Model file for the job. Use its own axes, mm. A direction names the side the tool comes from. Round coordinates to 2 decimals unless told otherwise and drop trailing zeros. Order: outer loops, then holes, each group sorted by start corner. A loop starts at its lowest first (then second) coordinate and runs counter-clockwise, first axis right, second up. Notation, with made-up numbers: (81, 14) -> (106, 14) arc R4 ccw to (106, 19) -> close; hole circle Ø3 at (25.5, -32). An arc over 180 degrees is marked (long way). Put each result on its own line as item: value. Start each with the question number.
Q1. Cut at B-B, the plane x = 10. List the corners of the cut face in (y, z).
Q2. Probe L1, parallel to Y at x = 12, z = 10.25; L2, parallel to X at y = -20.5, z = 5.5; L3, parallel to Y at x = 0.7, z = 6. List the from-to ranges inside material, lowest first.
Q3. Cut at D-D, the plane y = -15.5. List the corners of the cut face in (x, z).
Q4. 3-axis set-ups, long thin cutter, end or side, ignore diameter. For faces 4 (the face through (8.1, -0.5, 0)), 5 (the face through (1, -18, 6)): which of +Z, -Z, +X, -X, +Y, -Y reach the whole face in a straight line?
Q5. Cut at C-C, the plane z = 3.8. List the corners of the cut face in (x, y).
Q6. Cut at A-A, the plane y = -10. List the corners of the cut face in (x, z), and give its area (3 significant figures).
Q7. Pull direction Z, two halves, no side cores. Call faces 1 (the face through (8.1, -0.5, 12)), 2 (the face through (0.493, -11.464, 3.475)), 3 (the face through (18, -1, 6)): released by +Z, released by -Z, zero draft, split by the parting line, or undercut.
Q8. Flat gauge pins, fed straight in: P1, Ø6, axis at x = 21, z = 5, coming from the -Y side; P2, Ø4, axis at y = -10, z = 2.5, coming from the +X side; P3, Ø3, axis at y = -22, z = 2.5, coming from the -X side. Where does each tip first touch, or does it go through?
from build123d import *

# Parameters (mm, degrees)
EXTRUDE_1_DEPTH     = 12
FILLET_1_R          = 6
FILLET_2_R          = 2
FILLET_3_R          = 0.5
SKETCH_2_R          = 1.5
CUT_EXTRUDE_1_DEPTH = 51.931326313
SKETCH_3_R          = 1.5
CUT_EXTRUDE_2_DEPTH = 51.931326313


with BuildPart() as part:
    # 草图1 → 凸台-拉伸1 (new body)
    with BuildSketch(Plane.XY):
        Polygon((0, 0), (35, 0), (35, -1), (1, -1), (1, -35), (0, -35), align=None)
    extrude(amount=EXTRUDE_1_DEPTH)

    # 圆角1
    fillet_1_edges = [part.edges().sort_by_distance(p)[0] for p in [
        (0.5, -35, 12),
        (0.5, -35, 0),
        (35, -0.5, 0),
        (35, -0.5, 12),
    ]]
    fillet(fillet_1_edges, radius=FILLET_1_R - 0.0001)  # a hair under: the kernel refuses the full size

    # 圆角2
    fillet_2_edges = [part.edges().sort_by_distance(p)[0] for p in [
        (0, 0, 6),
    ]]
    fillet(fillet_2_edges, radius=FILLET_2_R)

    # 圆角3
    fillet_3_edges = [part.edges().sort_by_distance(p)[0] for p in [
        (1, -1, 6),
    ]]
    fillet(fillet_3_edges, radius=FILLET_3_R)

    # 草图2 → 切除-拉伸1 (cut, through all)
    with BuildSketch(Plane.ZY):
        with Locations((6, -29)):
            Circle(SKETCH_2_R)
        with Locations((3.8, -10)):
            Circle(SKETCH_2_R)
    extrude(amount=-CUT_EXTRUDE_1_DEPTH, mode=Mode.SUBTRACT)

    # 草图3 → 切除-拉伸2 (cut, through all)
    with BuildSketch(Plane(origin=(0, 0, 0), x_dir=(1, 0, 0), z_dir=(0, 1, 0))):
        with Locations(Location((29, -6, 0), (0, 0, 270))):
            Circle(SKETCH_3_R)
        with Locations(Location((10, -8.2, 0), (0, 0, 270))):
            Circle(SKETCH_3_R)
    extrude(amount=-CUT_EXTRUDE_2_DEPTH, mode=Mode.SUBTRACT)


solid = part.part
Ans:
1. outline: (-1, 0) -> (0, 0) -> (0, 6.7) -> (-1, 6.7) -> close; (-1, 9.7) -> (0, 9.7) -> (0, 12) -> (-1, 12) -> close
2. L1: y = -1 to 0
2. L2: x = 0 to 1
2. L3: y = -35 to -30.5, -27.5 to -0.48
3. outline: (0, 0) -> (1, 0) -> (1, 12) -> (0, 12) -> close
4. face 4: -Z, +X, -X, +Y, -Y
4. face 5: +Z, -Z, +X, -Y
5. outline: (0, -34.58) -> (1, -34.58) -> (1, -11.5) -> (0, -11.5) -> close; (0, -8.5) -> (1, -8.5) -> (1, -1.5) arc R0.5 cw to (1.5, -1) -> (34.58, -1) -> (34.58, 0) -> (2, 0) arc R2 ccw to (0, -2) -> close
6. outline: (0, 0) -> (1, 0) -> (1, 2.3) -> (0, 2.3) -> close; (0, 5.3) -> (1, 5.3) -> (1, 12) -> (0, 12) -> close
6. area: 9.00 mm^2
7. face 1: released by +Z
7. face 2: undercut
7. face 3: zero draft
8. P1: stops at y = -1
8. P2: stops at x = 1
8. P3: stops at x = 0
